```python
from build123d import *

# Parameters (mm, degrees)
SKETCH1_R           = 1.27
BOSS_EXTRUDE1_DEPTH = 6.35
SKETCH2_W           = 7.62
SKETCH2_H           = 58.928
BOSS_EXTRUDE2_DEPTH = 21.59
SKETCH3_R           = 1.905
BOSS_EXTRUDE3_DEPTH = 3.81
FILLET1_R           = 2.54


with BuildPart() as part:
    # Sketch1 → Boss-Extrude1 (new body)
    with BuildSketch(Plane.XY):
        Polygon((0, 0), (20.32, 0), (20.32, -7.62), (-7.62, -7.62), (-7.62, 51.308), (20.32, 51.308), (20.32, 43.688), (0, 43.688), align=None)
        with Locations((5.16001, 46.59376)):
            Circle(SKETCH1_R, mode=Mode.SUBTRACT)
        with Locations((15.15999, 46.59376)):
            Circle(SKETCH1_R, mode=Mode.SUBTRACT)
        with Locations((5.16001, -2.90576)):
            Circle(SKETCH1_R, mode=Mode.SUBTRACT)
        with Locations((15.15999, -2.90576)):
            Circle(SKETCH1_R, mode=Mode.SUBTRACT)
    extrude(amount=BOSS_EXTRUDE1_DEPTH)

    # Sketch2 → Boss-Extrude2 (add)
    with BuildSketch(Plane(origin=(0, 0, 0), x_dir=(-1, 0, 0), z_dir=(0, 0, -1))):
        with Locations((3.81, 21.844)):
            Rectangle(SKETCH2_W, SKETCH2_H)
    extrude(amount=BOSS_EXTRUDE2_DEPTH)

    # Sketch3 → Boss-Extrude3 (add)
    # profile 1 of 2: a face of its own
    with BuildSketch(Plane(origin=(0, 0, -21.59), x_dir=(-1, 0, 0), z_dir=(0, 0, -1))):
        with BuildLine():
            Line((13.97, 42.799), (7.62, 42.799))
            Line((7.62, 42.799), (7.62, 32.639))
            Line((7.62, 32.639), (13.97, 32.639))
            ThreePointArc((13.97, 32.639), (19.05, 37.719), (13.97, 42.799))
        make_face()
        with Locations((13.97, 37.719)):
            Circle(SKETCH3_R, mode=Mode.SUBTRACT)
    # profile 2 of 2: a face of its own
    with BuildSketch(Plane(origin=(0, 0, -21.59), x_dir=(-1, 0, 0), z_dir=(0, 0, -1))):
        with BuildLine():
            Line((13.97, 11.049), (7.62, 11.049))
            Line((7.62, 11.049), (7.62, 0.889))
            Line((7.62, 0.889), (13.97, 0.889))
            ThreePointArc((13.97, 0.889), (19.05, 5.969), (13.97, 11.049))
        make_face()
        with Locations((13.97, 5.969)):
            Circle(SKETCH3_R, mode=Mode.SUBTRACT)
    extrude(amount=-BOSS_EXTRUDE3_DEPTH)

    # Fillet1
    fillet1_edges = [part.edges().sort_by_distance(p)[0] for p in [
        (0, -3.81, 0),
        (0, 47.498, 0),
        (-7.62, 37.719, -17.78),
        (-7.62, 32.639, -19.685),
        (-7.62, 42.799, -19.685),
        (-7.62, 5.969, -17.78),
        (-7.62, 0.889, -19.685),
        (-7.62, 11.049, -19.685),
    ]]
    fillet(fillet1_edges, radius=FILLET1_R)


solid = part.part
```
Here's how the part is built. I have some questions about the finished solid (model axes, mm). A direction names the side the tool comes from. Round coordinates to 2 decimals unless told otherwise and drop trailing zeros. Loops run counter-clockwise (first coordinate to the right, second up) from the corner with the lowest first, then second, coordinate; pieces in that order, holes last.
1. Thinking about a two-plate mould opening in X: for faces 5 (the face through (20.32, -4, 3)), 6 (the face through (4.995, -1.647, 3.131)), 7 (the face through (-7.62, 21, -7)), 8 (the face through (-12, 42.799, -20)), which applies, released by +X, released by -X, zero draft, split by the parting line, or undercut?
Answers:
face 5: released by +X
face 6: undercut
face 7: released by -X
face 8: zero draft
2. Suppose I cut it at C-C, the plane z = -9.5. Please give me the cut outline in (x, y).
Answers:
outline: (-7.62, -7.62) - (0, -7.62) - (0, 51.31) - (-7.62, 51.31) - close
3. Suppose I cut it at A-A, the plane x = 10.5. Please give me the cut outline in (y, z).
Answers:
outline: (-7.62, 0) - (0, 0) - (0, 6.35) - (-7.62, 6.35) - close; (43.69, 0) - (51.31, 0) - (51.31, 6.35) - (43.69, 6.35) - close
4. If I drill on probe 1 along Y at (x, z) = (-13.97, -19.25); probe 2 along X at (y, z) = (10.5, -7); probe 3 along Z at (x, y) = (14, -0.5), over which ranges is the centre line in solid material (lowest first)?
Answers:
probe 1: y = 0.89 to 4.06, 7.87 to 11.05, 32.64 to 35.81, 39.62 to 42.8
probe 2: x = -7.62 to 0
probe 3: z = 0 to 6.35
5. Will these pins go through, and if not, where does the flat tip stop? pin 1 (3 mm diameter, centred on y = 41.5, z = -2.5, fed in from -X); pin 2 (10 mm diameter, centred on x = -16, y = 5, fed in from +Z); pin 3 (6 mm diameter, centred on x = 12, y = -5.5, fed in from -Z); pin 4 (4 mm diameter, centred on x = 5.16, y = -2.91, fed in from +Z).
Answers:
pin 1: stops at x = -7.62
pin 2: stops at z = -17.78
pin 3: stops at z = 0
pin 4: stops at z = 6.35
6. Suppose I cut it at B-B, the plane z = 4.5. Please give me the cut outline in (x, y), and give its area (3 significant figures).
Answers:
outline: (-7.62, -7.62) - (20.32, -7.62) - (20.32, 0) - (0, 0) - (0, 43.69) - (20.32, 43.69) - (20.32, 51.31) - (-7.62, 51.31) - close; hole circle Ø2.54 at (5.16, -2.91); hole circle Ø2.54 at (5.16, 46.59); hole circle Ø2.54 at (15.16, -2.91); hole circle Ø2.54 at (15.16, 46.59)
area: 738 mm2
7. Suppose I cut it at D-D, the plane y = 3. Please give me the cut outline in (x, z), and give its area (3 significant figures).
Answers:
outline: (-18.09, -21.59) - (0, -21.59) - (0, 6.35) - (-7.62, 6.35) - (-7.62, -15.24) arc R2.54 cw to (-10.16, -17.78) - (-18.09, -17.78) - close
area: 254 mm2
8. For faces 1 (the face through (-12, 0.889, -20)), 2 (the face through (-16, 7, -17.78)), 3 (the face through (-8.344, 31.875, -19.076)), 4 (the face through (12, -4, 0)), which set-ups out of +Z, -Z, +X, -X, +Y, -Y let a thin tool reach every point of the face, with its end or its side?
Answers:
face 1: +Z, -Z, -X, -Y
face 2: +Z, -X, +Y, -Y
face 3: +Z, -Z, -X
face 4: -Z, +X, +Y, -Y
